Design review of the part built by this model. Coordinates are the model's own, in mm. A direction names the side the tool comes from. Coordinates: 2 decimals unless noted, no trailing zeros. Write each loop counter-clockwise with the first axis right and the second up, starting at its lowest first coordinate (ties: lowest second). Pieces come first, ordered by that corner, then holes. Notation, with made-up numbers: (71.25, 59) -> (104.25, 59) arc R27 ccw to (104.25, 81) -> close; hole circle Ø5 at (30.5, -28.75). An arc over 180 degrees is marked (long way). Write item = value, one per line. Start each with the question number.
```python
from build123d import *

# Parameters (mm, degrees)
F0_W      = 1020
F0_H      = 17.9999992251
F1_DEPTH  = 280
F2_DEPTH  = 280
F3_W      = 280
F3_H      = 795.9999984503
F4_DEPTH  = 18
F5_W      = 280
F5_H      = 795.9999984503
F6_DEPTH  = 18
F7_W      = 1091.9999984503
F7_H      = 280
F8_DEPTH  = 18
F9_W      = 18
F9_H      = 795.9999984503
F10_DEPTH = 21
F11_DEPTH = 21
F12_DEPTH = 21
F14_DEPTH = 100
F15_W     = 508.5
F15_H     = 760
F16_DEPTH = 18
F17_DEPTH = 18
F18_R     = 15
F19_DEPTH = 30
F20_R     = 20
F20_R_2   = 15
F21_DEPTH = 10


with BuildPart() as f1:
    # F0 (on Front) → F1 (new body)
    with BuildSketch(Plane.XZ):
        with Locations((0, 388.9999996126)):
            Rectangle(F0_W, F0_H)
    extrude(amount=-F1_DEPTH)

    # F0 (on Front) → F2 (join)
    with BuildSketch(Plane.XZ):
        Polygon((510, -397.9999992251), (527.9999992251, -397.9999992251), (527.9999992251, 397.9999992251), (510, 397.9999992251), (510, 380), (510, -380), align=None)
        with Locations((0, -388.9999996126)):
            Rectangle(F0_W, F0_H)
        Polygon((-527.9999992251, -397.9999992251), (-510, -397.9999992251), (-510, -380), (-510, 380), (-510, 397.9999992251), (-527.9999992251, 397.9999992251), align=None)
        with Locations((0, 388.9999996126)):
            Rectangle(F0_W, F0_H)
    extrude(amount=-F2_DEPTH)

    # F3 (on face) → F4 (join)
    with BuildSketch(Plane.YZ.offset(527.9999992251)):
        with Locations((140, 0)):
            Rectangle(F3_W, F3_H)
    extrude(amount=F4_DEPTH)

    # F5 (on face) → F6 (join)
    with BuildSketch(Plane(origin=(-527.9999992251, 0, 0), x_dir=(0, -1, 0), z_dir=(-1, 0, 0))):
        with Locations((-140, 0)):
            Rectangle(F5_W, F5_H)
    extrude(amount=F6_DEPTH)

    # F7 (on face) → F8 (join)
    with BuildSketch(Plane.XY.offset(397.9999992251)):
        with Locations((0, 140)):
            Rectangle(F7_W, F7_H)
        Polygon((553.9999992251, 280), (545.9999992251, 280), (545.9999992251, 0), (-545.9999992251, 0), (-545.9999992251, -30), (553.9999992251, -30), align=None)
    extrude(amount=F8_DEPTH)

    # F9 (on face) → F10 (join)
    with BuildSketch(Plane.XZ):
        with Locations((-536.9999992251, 0)):
            Rectangle(F9_W, F9_H)
    extrude(amount=F10_DEPTH)

    # F9 (on face) → F11 (join)
    with BuildSketch(Plane.XZ):
        with Locations((536.9999992251, 0)):
            Rectangle(F9_W, F9_H)
    extrude(amount=F11_DEPTH)

    # F12 (add): a face of the model
    f12_faces = [f1.faces().sort_by_distance(p)[0] for p in [
        (4, -30, 406.9999992251),
    ]]
    extrude(f12_faces, amount=F12_DEPTH)

    # F13 (on face) → F14 (join)
    with BuildSketch(Plane(origin=(0, 0, -397.9999992251), x_dir=(1, 0, 0), z_dir=(0, 0, -1))):
        Polygon((-495.9999992251, -50), (-495.9999992251, -280), (-476.9999992251, -280), (-476.9999992251, -69), (476.9999992251, -69), (476.9999992251, -280), (495.9999992251, -280), (495.9999992251, -50), align=None)
    extrude(amount=F14_DEPTH)

    # F15 (on face) → F16 (join)
    with BuildSketch(Plane.XZ):
        Polygon((-1.5, 380), (-1.5, 394.9999992251), (-524.9999992251, 394.9999992251), (-524.9999992251, -394.9999992251), (-1.5, -394.9999992251), (-1.5, -380), (-510, -380), (-510, 380), align=None)
        with Locations((-255.75, 0)):
            Rectangle(F15_W, F15_H)
    extrude(amount=F16_DEPTH)

    # F15 (on face) → F17 (join)
    with BuildSketch(Plane.XZ):
        Polygon((524.9999992251, -394.9999992251), (524.9999992251, 394.9999992251), (1.5, 394.9999992251), (1.5, 380), (510, 380), (510, -380), (1.5, -380), (1.5, -394.9999992251), align=None)
        with Locations((255.75, 0)):
            Rectangle(F15_W, F15_H)
    extrude(amount=F17_DEPTH)

    # F18 (on face) → F19 (join)
    with BuildSketch(Plane.XZ.offset(18)):
        with Locations((-51.5, 344.9999992251)):
            Circle(F18_R)
    extrude(amount=F19_DEPTH)

    # F20 (on face) → F21 (join)
    with BuildSketch(Plane.XZ.offset(48)):
        with Locations((-51.5, 344.9999992251)):
            Circle(F20_R)
        with Locations((-51.5, 344.9999992251)):
            Circle(F20_R_2, mode=Mode.SUBTRACT)
    extrude(amount=-F21_DEPTH)

    # F22: F1 across plane


with BuildPart() as f1_1:
    add(f1.part)
    add(f1.part.mirror(Plane.YZ))


solid = f1_1.part
```
(1) Take a section at A-A, the plane y = 130. State the section outline as (x, z) points.
(2) For line 1 (Z direction, x = 419, y = 250); line 2 (X direction, y = 180.5, z = -184.5); line 3 (Y direction, x = -122, z = -325.5), list the stretches that pass through material, from the lowest coordinate up.
(3) Take a section at C-C, the plane z = -411.5. State the section outline as (x, y) points, then the cut area to 3 significant figures.
(4) Take a section at B-B, the plane z = -86.5. State the section outline as (x, y) points, then the cut area to 3 significant figures.
(5) Mouldability with a two-part tool opening along X and no side actions: class faces 6 (the face through (546, 132, -6)), 7 (the face through (-259, 0, 5)), 8 (the face through (-3, 41, -398)) as pulls with the +X half, pulls with the -X half, needs draft (parallel to the pull), parting line crosses it, or undercut.
(6) For faces 1 (the face through (-7, 69, -447)), 2 (the face through (-510, 138, -5)), 3 (the face through (-53.453, -27.86, 359.872)), 4 (the face through (55.836, -43.07, 325.476)), 5 (the face through (496, 167, -447)), list the 3-axis set-ups (+Z, -Z, +X, -X, +Y, -Y) from which the entire face can be reached by the end or side of a thin tool; tool diameter is ignored.
(7) For pin 1 Ø14.5 at (y, z) = (-12.5, 156) entering from -X; pin 2 Ø5 at (x, z) = (441.5, 17.5) entering from +Y; pin 3 Ø9 at (x, y) = (200, -8) entering from -Z, all flat-tipped, find the tip position at first contact; note any pin that passes through.
(8) Take a section at D-D, the plane x = 51.5. State the section outline as (y, z) points, then the cut area to 3 significant figures.
Report:
q1.outline = (-554, 398) -> (-546, 398) -> (-546, -398) -> (-496, -398) -> (-496, -498) -> (-477, -498) -> (-477, -398) -> (477, -398) -> (477, -498) -> (496, -498) -> (496, -398) -> (546, -398) -> (546, 398) -> (554, 398) -> (554, 416) -> (-554, 416) -> close; hole (-510, -380) -> (510, -380) -> (510, 380) -> (-510, 380) -> close
q2.line_1 = -398 to -380, 380 to 416
q2.line_2 = -546 to -510, 510 to 546
q2.line_3 = -18 to 0
q3.outline = (-496, 50) -> (496, 50) -> (496, 280) -> (477, 280) -> (477, 69) -> (-477, 69) -> (-477, 280) -> (-496, 280) -> close
q3.area = 26,900 mm2
q4.outline = (-546, -21) -> (-528, -21) -> (-528, 0) -> (-525, 0) -> (-525, -18) -> (-1.5, -18) -> (-1.5, 0) -> (-510, 0) -> (-510, 280) -> (-546, 280) -> close; (1.5, -18) -> (525, -18) -> (525, 0) -> (528, 0) -> (528, -21) -> (546, -21) -> (546, 280) -> (510, 280) -> (510, 0) -> (1.5, 0) -> close
q4.area = 39,800 mm2
q5.face_6 = pulls with the +X half
q5.face_7 = undercut
q5.face_8 = needs draft
q6.face_1 = -Z, +Y
q6.face_2 = +Y
q6.face_3 = none
q6.face_4 = -Y
q6.face_5 = -Z, +X, +Y, -Y
q7.pin_1 = -546
q7.pin_2 = 0
q7.pin_3 = -395
q8.outline = (-51, 398) -> (0, 398) -> (0, 395) -> (-18, 395) -> (-18, 360) -> (-38, 360) -> (-38, 365) -> (-48, 365) -> (-48, 325) -> (-38, 325) -> (-38, 330) -> (-18, 330) -> (-18, -395) -> (0, -395) -> (0, -398) -> (50, -398) -> (50, -498) -> (69, -498) -> (69, -398) -> (280, -398) -> (280, -380) -> (0, -380) -> (0, 380) -> (280, 380) -> (280, 416) -> (-51, 416) -> close
q8.area = 33,200 mm2
